The model under review builds one solid part; all positions refer to its coordinate system, in mm. A direction names the side the tool comes from. Coordinates: 2 decimals unless noted, no trailing zeros. Order: outer loops, then holes, each group sorted by start corner. A loop starts at its lowest first (then second) coordinate and runs counter-clockwise, first axis right, second up. Notation, with made-up numbers: (79, -17.75) -> (86, -17.75) arc R22 ccw to (86, 13.25) -> close; hole circle Ø8 at (34.25, 51.5). An arc over 180 degrees is marked (long way). Use one line per item in the form item = value.
from build123d import *

# Parameters (mm, degrees)
SKETCH1_R           = 12.5
SKETCH1_R_2         = 11.25
BOSS_EXTRUDE1_DEPTH = 210
SKETCH2_R           = 22.5
SKETCH2_R_2         = 11.25
BOSS_EXTRUDE2_DEPTH = 3
BOSS_EXTRUDE3_START = 3
SKETCH3_R           = 15
SKETCH3_R_2         = 11.25
BOSS_EXTRUDE3_DEPTH = 3


with BuildPart() as part:
    # Sketch1 → Boss-Extrude1 (new, symmetric)
    with BuildSketch(Plane(origin=(0, 0, 0), x_dir=(1, 0, 0), z_dir=(0, 1, 0))):
        with Locations(Location((0, 0, 0), (0, 0, 270))):
            Circle(SKETCH1_R)
        with Locations(Location((0, 0, 0), (0, 0, 270))):
            Circle(SKETCH1_R_2, mode=Mode.SUBTRACT)
    extrude(amount=BOSS_EXTRUDE1_DEPTH, both=True)

    # Sketch2 → Boss-Extrude2 (add)
    with BuildSketch(Plane(origin=(0, 210, 0), x_dir=(1, 0, 0), z_dir=(0, 1, 0))):
        with Locations(Location((0, 0, 0), (0, 0, 270))):
            Circle(SKETCH2_R)
        with Locations(Location((0, 0, 0), (0, 0, 270))):
            Circle(SKETCH2_R_2, mode=Mode.SUBTRACT)
    extrude(amount=BOSS_EXTRUDE2_DEPTH)

    # Sketch3 → Boss-Extrude3 (add)
    with BuildSketch(Plane(origin=(0, -118, 0), x_dir=(-1, 0, 0), z_dir=(0, -1, 0)).offset(BOSS_EXTRUDE3_START)):
        with Locations(Location((0, 0, 0), (0, 0, 90))):
            Circle(SKETCH3_R)
        with Locations(Location((0, 0, 0), (0, 0, 270))):
            Circle(SKETCH3_R_2, mode=Mode.SUBTRACT)
    extrude(amount=-BOSS_EXTRUDE3_DEPTH)


solid = part.part
Item 1: To check wall thickness, follow L1, parallel to Z at x = -1, y = -10; L2, parallel to X at y = -41, z = 0; L3, parallel to Y at x = -10, z = -11. State the ranges of each line that lie inside material, in increasing order. Write a range as from..to.
Results found:
L1 = -12.46..-11.21, 11.21..12.46
L2 = -12.5..-11.25, 11.25..12.5
L3 = -121..-118, 210..213
Item 2: Draft analysis for pull direction Z (two halves, no side actions). For faces 1 (the face through (-4.31, -1.46, 10.39)), 2 (the face through (3.755, -164.877, 11.923)), 3 (the face through (-10, 210, 10)), state which applies: released by +Z, released by -Z, zero draft, split by the parting line, or undercut.
Results found:
face_1 = undercut
face_2 = split by the parting line
face_3 = zero draft
Item 3: We need section B-B (z = 0). Write out the cut boundary in (x, y).
Results found:
outline = (-22.5, 210) -> (-12.5, 210) -> (-12.5, -118) -> (-15, -118) -> (-15, -121) -> (-12.5, -121) -> (-12.5, -210) -> (-11.25, -210) -> (-11.25, 213) -> (-22.5, 213) -> close; (11.25, -210) -> (12.5, -210) -> (12.5, -121) -> (15, -121) -> (15, -118) -> (12.5, -118) -> (12.5, 210) -> (22.5, 210) -> (22.5, 213) -> (11.25, 213) -> close
Item 4: We need section C-C (y = 174). Write out the cut boundary in (x, z), plus the area to 3 significant figures.
Results found:
outline = circle Ø25 at (0, 0); hole circle Ø22.5 at (0, 0)
area = 93.3 mm²
Item 5: Tool access review of faces 4 (the face through (7, -210, -9)), 5 (the face through (12.3, -118, 3.4)), 6 (the face through (0.66, -119.521, 14.985)): name each direction out of +Z, -Z, +X, -X, +Y, -Y from which nothing blocks a thin tool from reaching the whole face with its end or side.
Results found:
face_4 = +Z, -Z, +X, -X, -Y
face_5 = none
face_6 = -Y
Item 6: We need section A-A (x = 0). Write out the cut boundary in (y, z), plus the area to 3 significant figures.
Results found:
outline = (-210, -12.5) -> (-121, -12.5) -> (-121, -15) -> (-118, -15) -> (-118, -12.5) -> (210, -12.5) -> (210, -22.5) -> (213, -22.5) -> (213, -11.25) -> (-210, -11.25) -> close; (-210, 11.25) -> (213, 11.25) -> (213, 22.5) -> (210, 22.5) -> (210, 12.5) -> (-118, 12.5) -> (-118, 15) -> (-121, 15) -> (-121, 12.5) -> (-210, 12.5) -> close
area = 1,130 mm²
Item 7: Clearance check with flat-ended pins moving along their axes: pin 1 (6 mm diameter, centred on y = -80, z = 12.5, fed in from -X); pin 2 (10 mm diameter, centred on y = 17.5, z = 3, fed in from +X); pin 3 (5 mm diameter, centred on x = -15.5, y = -154, fed in from -Z); pin 4 (6 mm diameter, centred on x = -13.5, y = -13.5, fed in from -Z). State where each tip first meets the part, or that it passes through.
Results found:
pin_1 = -8.12
pin_2 = 12.5
pin_3 = through
pin_4 = -6.78
Item 8: We need section D-D (z = 19). Write out the cut boundary in (x, y).
Results found:
outline = (-12.05, 210) -> (12.05, 210) -> (12.05, 213) -> (-12.05, 213) -> close
